```python
from build123d import *

# Parameters (mm, degrees)
SKETCH_2_W                  = 8
SKETCH_2_H                  = 37
SM_BASE_FLANGE_1_DEPTH      = 2
SM_EDGE_FLANGE_1_DEPTH      = 14
SM_START                    = 2
SM_EDGE_FLANGE_1_FLAT_DEPTH = 2
HOLE_WIZARD_M5_2_D          = 5.5
CUT_EXTRUDE_1_DEPTH         = 28.555654592
CUT_EXTRUDE_1_DEPTH_BACK    = 28.555654592


# Sheet-metal steps are written as plain solids
with BuildPart() as part:
    # Sketch 2 → 基体-法兰1 (new body)
    with BuildSketch(Plane(origin=(0, 0, 0), x_dir=(1, 0, 0), z_dir=(0, 1, 0))):
        Rectangle(SKETCH_2_W, SKETCH_2_H)
    extrude(amount=-SM_BASE_FLANGE_1_DEPTH)

    # 边线-法兰1 bend section (across the edge) → 边线-法兰1 (add)
    with BuildSketch(Plane(origin=(-6, 0, -18.5), x_dir=(1, 0, 0), z_dir=(0, 0, 1))):
        with BuildLine():
            Line((-2, 2), (0, 2))
            ThreePointArc((0, 2), (0.585786438, 0.585786438), (2, 0))
            Line((2, 0), (2, -2))
            ThreePointArc((2, -2), (-0.828427125, -0.828427125), (-2, 2))
        make_face()
    sm_edge_flange_1 = extrude(amount=SM_EDGE_FLANGE_1_DEPTH)

    # 边线-法兰1 profile (on flange) → 边线-法兰1 flat (add)
    with BuildSketch(Plane.ZY.offset(6).offset(SM_START)):
        with BuildLine():
            ThreePointArc((-4.5, 11.79), (-11.5, 18.79), (-18.5, 11.79))
            Line((-18.5, 11.79), (-18.5, 2))
            Line((-18.5, 2), (-4.5, 2))
            Line((-4.5, 2), (-4.5, 11.79))
        make_face()
    sm_edge_flange_1_flat = extrude(amount=-SM_EDGE_FLANGE_1_FLAT_DEPTH)

    # 镜向1: 边线-法兰1, 边线-法兰1 flat across plane
    add(sm_edge_flange_1.mirror(Plane(origin=(0, 0, 0), x_dir=(0, 0, 1), z_dir=(1, 0, 0))))
    add(sm_edge_flange_1_flat.mirror(Plane(origin=(0, 0, 0), x_dir=(0, 0, 1), z_dir=(1, 0, 0))))

    # M5 间隙孔2 (through all)
    with Locations(Plane.ZY.offset(8)):
        with Locations((-11.5, 11.79)):
            Hole(HOLE_WIZARD_M5_2_D / 2)

    # 草图22 → 切除-拉伸1 (cut, two sides: drawn at the far end of the back side and taken through both)
    with BuildSketch(Plane(origin=(0, 0, 0), x_dir=(1, 0, 0), z_dir=(0, 1, 0)).offset(-CUT_EXTRUDE_1_DEPTH_BACK)):
        Polygon((88.803072858, -41.222914888), (4, -18.5), (-4, -16.356406461), (-88.803072858, 6.366508427), (-134.248902633, -163.239637288), (43.357243082, -210.829060603), align=None)
    extrude(amount=CUT_EXTRUDE_1_DEPTH + CUT_EXTRUDE_1_DEPTH_BACK, mode=Mode.SUBTRACT)


solid = part.part
```
Design review of the part built by this model. Coordinates are the model's own, in mm. A direction names the side the tool comes from. Give positions to 0.01 mm unless a question says otherwise; leave off trailing zeros. Loops run counter-clockwise (first coordinate to the right, second up) from the corner with the lowest first, then second, coordinate; pieces in that order, holes last. Notation, with made-up numbers: M 40.5,-37.5 L 83.5,-37.5 A17 ccw 83.5,-7.5 Z; hole C -3.75,6.5 d1. An arc over 180 degrees is marked long. Return JSON: item names as keys, results as strings. Group by question number.
Item 1: We need section C-C (z = -5.5). Give the boundary of the cut face in (x, y).
Item 2: Insertion check: pin 1 Ø2 at (x, y) = (6.5, 7) entering from +Z; pin 2 Ø5 at (x, z) = (3, 2) entering from +Y; pin 3 Ø0.6 at (y, z) = (-0.5, 4) entering from -X. Each pin has a flat end and moves straight along its axis. Give the tip position at first contact, or say it passes through.
Item 3: For probe 1 along X at (y, z) = (7.25, -10.5); probe 2 along Y at (x, z) = (2, 4.5); probe 3 along Y at (x, z) = (6.85, -11.5), list the stretches that pass through material, from the lowest coordinate up.
Item 4: We need section B-B (z = -11.5). Give the boundary of the cut face in (x, y).
Item 5: We need section A-A (y = 6). Give the boundary of the cut face in (x, z).
Item 6: We need section D-D (x = 7.25). Give the boundary of the cut face in (y, z), and give its area (3 significant figures).
Item 7: Tool access review of faces 4 (the cylindrical face through (-6.797, -0.859, -11.598)), 5 (the flat face through (6, 8.6, -11.6)), 6 (the flat face through (4, -1, 7)), 7 (the flat face through (-4, -1, 6)): name each direction out of +Z, -Z, +X, -X, +Y, -Y from which nothing blocks a thin tool from reaching the whole face with its end or side.
Item 8: Mouldability with a two-part tool opening along Y and no side actions: class faces 1 (the cylindrical face through (-5.43, 0.6, -11.6)), 2 (the cylindrical face through (-6.986, 9.105, -10.904)), 3 (the flat face through (-8, 8.6, -11.6)) as released by +Y, released by -Y, zero draft, split by the parting line, or undercut.
Output:
{
 "1": {"outline": "M -8,2 A4 ccw -4,-2 L 4,-2 A4 ccw 8,2 L 8,15.4 L 6,15.4 L 6,2 A2 cw 4,0 L -4,0 A2 cw -6,2 L -6,15.4 L -8,15.4 Z"},
 "2": {"pin 1": "stops at z = -4.5", "pin 2": "stops at y = 0", "pin 3": "stops at x = -4"},
 "3": {"probe 1": "x = -8 to -6, 6 to 8", "probe 2": "y = -2 to 0", "probe 3": "y = -0.81 to 9.04, 14.54 to 18.79"},
 "4": {"outline": "M -8,2 A4 ccw -4,-2 L 4,-2 A4 ccw 8,2 L 8,9.04 L 6,9.04 L 6,2 A2 cw 4,0 L -4,0 A2 cw -6,2 L -6,9.04 L -8,9.04 Z; M -8,14.54 L -6,14.54 L -6,18.79 L -8,18.79 Z; M 6,14.54 L 8,14.54 L 8,18.79 L 6,18.79 Z"},
 "5": {"outline": "M -8,-18.5 L -6,-18.5 L -6,-4.5 L -8,-4.5 Z; M 6,-18.5 L 8,-18.5 L 8,-4.5 L 6,-4.5 Z"},
 "6": {"outline": "M -0.33,-18.5 L 11.79,-18.5 A7 ccw 11.79,-4.5 L -0.33,-4.5 Z; hole C 11.79,-11.5 d5.5", "area": "223 mm^2"},
 "7": {"face 4": "+Z, -Z, -X, -Y", "face 5": "+Z, -Z, +Y", "face 6": "+Z, +X, +Y, -Y", "face 7": "+Z, -X, +Y, -Y"},
 "8": {"face 1": "released by +Y", "face 2": "undercut", "face 3": "zero draft"}
}
